from build123d import *

# Parameters (mm, degrees)
F1_DEPTH = 50.8


with BuildPart() as f1:
    # F0 (on Front) → F1 (new body)
    with BuildSketch(Plane.XZ):
        with BuildLine():
            Line((157.3511064053, 226.7855703831), (117.0178577304, 256.9078505039))
            Line((117.0178577304, 256.9078505039), (153.2667279243, 222.1906334162))
            Line((153.2667279243, 222.1906334162), (135.5471188815, 203.6892712114))
            ThreePointArc((135.5471188815, 203.6892712114), (124.4679795229, 189.3777542773), (142.5452232361, 188.4945183992))
            Line((142.5452232361, 188.4945183992), (157.3511064053, 188.4945183992))
            ThreePointArc((157.3511064053, 188.4945183992), (163.0913283676, 173.9439144731), (157.3511064053, 159.3933105469))
            ThreePointArc((157.3511064053, 159.3933105469), (133.5218764448, 146.628732852), (106.8485764131, 151.0221039559))
            ThreePointArc((106.8485764131, 151.0221039559), (81.4826477265, 155.0355463169), (59.0786326768, 142.4817354462))
            ThreePointArc((59.0786326768, 142.4817354462), (57.1778936646, 140.1694279188), (55.4591871163, 137.7187907169))
            ThreePointArc((55.4591871163, 137.7187907169), (49.1972996165, 115.7594263547), (56.2388920861, 94.0375274104))
            ThreePointArc((56.2388920861, 94.0375274104), (51.4005357949, 84.435997918), (44.5201359689, 76.1740878224))
            ThreePointArc((44.5201359689, 76.1740878224), (33.1757105593, 71.4588467738), (31.2459021807, 59.3260265887))
            ThreePointArc((31.2459021807, 59.3260265887), (28.0144474885, 44.7267728634), (21.5454995632, 31.2459263951))
            ThreePointArc((21.5454995632, 31.2459263951), (25.0258299967, 19.4454210796), (26.6509782523, 7.2501958348))
            Line((26.6509782523, 7.2501958348), (45.5412305892, 7.2501958348))
            ThreePointArc((45.5412305892, 7.2501958348), (43.9865002742, 15.1994537749), (37.8830172122, 20.52443102))
            ThreePointArc((37.8830172122, 20.52443102), (39.9724122876, 31.2459263951), (37.8830172122, 41.9674217701))
            ThreePointArc((37.8830172122, 41.9674217701), (43.3657124777, 53.2576823746), (51.4005357949, 62.8998577595))
            ThreePointArc((51.4005357949, 62.8998577595), (63.9434482796, 70.1826306752), (75.6635218859, 78.7268280983))
            ThreePointArc((75.6635218859, 78.7268280983), (79.7479003668, 78.2162845135), (83.8322788477, 78.7268280983))
            ThreePointArc((83.8322788477, 78.7268280983), (80.62219761, 70.8415194676), (75.6635218859, 63.9209523797))
            ThreePointArc((75.6635218859, 63.9209523797), (94.8811032097, 51.3116760169), (110.8912838002, 34.8197567898))
            Line((110.8912838002, 34.8197567898), (118.0389523506, 23.5877130181))
            ThreePointArc((118.0389523506, 23.5877130181), (122.7991958663, 28.8657998516), (124.165520072, 35.8408465981))
            ThreePointArc((124.165520072, 35.8408465981), (117.7349645729, 43.3549786498), (114.4651249051, 52.6889152825))
            ThreePointArc((114.4651249051, 52.6889152825), (101.2536184714, 56.1015596962), (93.0221304297, 66.9842362404))
            ThreePointArc((93.0221304297, 66.9842362404), (105.7958752022, 76.2573128263), (114.4651249051, 89.4483178854))
            ThreePointArc((114.4651249051, 89.4483178854), (137.6729881459, 85.3431639936), (161.1937859731, 86.8362394266))
            Line((161.1937859731, 86.8362394266), (161.1937859731, 60.947837063))
            add(Edge.make_bspline(
                [(161.1937859731, 60.947837063), (157.8993693687, 59.0561358776), (150.6323180509, 54.8832909577), (162.2144334117, 39.9763215602), (143.2040633117, 24.6385665246), (159.3573781955, 18.7003155427), (150.8482458466, 9.9391907933), (152.7499995265, 7.8050355296)],
                knots=[0, 0, 0, 0, 0.0779334272, 0.1719109278, 0.2757758884, 0.3531240541, 0.4319815568, 0.4319815568, 0.4319815568, 0.4319815568], degree=3))
            Line((152.7499995265, 7.8050355296), (173.171891931, 9.0224858617))
            ThreePointArc((173.171891931, 9.0224858617), (172.9779809567, 10.1232568284), (172.664853356, 11.1962196856))
            add(Edge.make_bspline(
                [(172.664853356, 11.1962196856), (171.3313436819, 12.7085104711), (168.5824067748, 14.597468285), (167.0453242097, 17.1912484114)],
                knots=[0.5736467919, 0.5736467919, 0.5736467919, 0.5736467919, 0.6257117477, 0.6257117477, 0.6257117477, 0.6257117477], degree=3))
            add(Edge.make_bspline(
                [(167.0453242097, 17.1912484114), (166.5426299969, 18.0395296218), (166.169553332, 18.9631972351), (165.9011092746, 19.9468993754)],
                knots=[0.6257117477, 0.6257117477, 0.6257117477, 0.6257117477, 0.6427392989, 0.6427392989, 0.6427392989, 0.6427392989], degree=3))
            ThreePointArc((165.9011092746, 19.9468993754), (164.2768081704, 31.0782012829), (167.0453242097, 41.9813914203))
            add(Edge.make_bspline(
                [(167.0453242097, 41.9813914203), (167.3962963394, 49.2992780507), (165.4846355858, 55.0477309675), (167.0453242097, 61.3542387283)],
                knots=[0.7506807864, 0.7506807864, 0.7506807864, 0.7506807864, 0.8611546748, 0.8611546748, 0.8611546748, 0.8611546748], degree=3))
            add(Edge.make_bspline(
                [(167.0453242097, 61.3542387283), (169.0068222846, 69.2803571375), (176.4531944079, 78.0879710988), (183.8995665312, 86.8955850601)],
                knots=[0.8611546748, 0.8611546748, 0.8611546748, 0.8611546748, 1, 1, 1, 1], degree=3))
            ThreePointArc((183.8995665312, 86.8955850601), (200.6813055662, 83.248064902), (217.7208593273, 85.3892738977))
            ThreePointArc((217.7208593273, 85.3892738977), (229.8786920932, 81.8087152157), (231.4277632013, 69.2296183983))
            Line((231.4277632013, 69.2296183983), (228.5562352695, 63.4104087949))
            Line((228.5562352695, 63.4104087949), (231.4277632013, 57.001966241))
            Line((231.4277632013, 57.001966241), (221.0727564471, 52.3620415043))
            Line((221.0727564471, 52.3620415043), (222.7011620998, 44.7454368664))
            Line((222.7011620998, 44.7454368664), (237.3357014598, 47.8742544631))
            Line((237.3357014598, 47.8742544631), (240.5703216791, 63.4104087949))
            Line((240.5703216791, 63.4104087949), (240.5703216791, 81.790111959))
            ThreePointArc((240.5703216791, 81.790111959), (237.5070340931, 96.5959839523), (222.7011620998, 99.6592715383))
            Line((222.7011620998, 99.6592715383), (208.9163959026, 107.8280285001))
            ThreePointArc((208.9163959026, 107.8280285001), (216.2226754166, 127.6019199845), (215.5535072088, 148.6718207598))
            ThreePointArc((215.5535072088, 148.6718207598), (218.0854842896, 143.9483475476), (222.190618515, 140.503063798))
            ThreePointArc((222.190618515, 140.503063798), (220.0514151702, 151.3432226251), (215.5535072088, 161.4354997873))
            Line((215.5535072088, 161.4354997873), (229.0830209851, 152.8838410974))
            Line((229.0830209851, 152.8838410974), (214.0218615532, 172.6675480604))
            Line((214.0218615532, 172.6675480604), (219.6378856897, 172.6675480604))
            Line((219.6378856897, 172.6675480604), (208.4058374166, 184.6981031667))
            Line((208.4058374166, 184.6981031667), (213.5113179684, 186.4523291588))
            Line((213.5113179684, 186.4523291588), (208.4058374166, 201.3112651118))
            Line((208.4058374166, 201.3112651118), (213.5113179684, 201.7687410116))
            Line((213.5113179684, 201.7687410116), (200.6355195315, 214.0218764544))
            Line((200.6355195315, 214.0218764544), (208.4058374166, 213.5113328695))
            ThreePointArc((208.4058374166, 213.5113328695), (200.6355195315, 219.8232430535), (191.0472214222, 222.7011919022))
            ThreePointArc((191.0472214222, 222.7011919022), (182.6973201136, 228.8132361759), (172.5500786904, 226.7855703831))
            Line((172.5500786904, 226.7855703831), (167.7524379956, 231.3804924488))
            Line((167.7524379956, 231.3804924488), (167.7524379956, 226.7855703831))
            Line((167.7524379956, 226.7855703831), (161.0753406305, 231.77226012))
            Line((161.0753406305, 231.77226012), (157.3511064053, 226.7855703831))
        make_face()
        with BuildLine():
            ThreePointArc((55.4591871163, 137.7187907169), (57.1778936646, 140.1694279188), (59.0786326768, 142.4817354462))
            ThreePointArc((59.0786326768, 142.4817354462), (39.0356978447, 161.9894984881), (18.9927630126, 142.4817354462))
            ThreePointArc((18.9927630126, 142.4817354462), (15.5809128086, 125.4101537656), (18.9927630126, 108.3385720849))
            Line((18.9927630126, 108.3385720849), (22.309999913, 97.1100777388))
            Line((22.309999913, 97.1100777388), (22.309999913, 84.7518071532))
            Line((22.309999913, 84.7518071532), (33.4528027138, 104.264870286))
            Line((33.4528027138, 104.264870286), (33.4528027138, 86.6916491587))
            Line((33.4528027138, 86.6916491587), (36.9130928491, 112.466349486))
            Line((36.9130928491, 112.466349486), (43.123934418, 97.1100777388))
            ThreePointArc((43.123934418, 97.1100777388), (41.9493193566, 113.4261599819), (37.8830172122, 129.2710155249))
            ThreePointArc((37.8830172122, 129.2710155249), (41.7069327363, 143.8231946906), (55.4591871163, 137.7187907169))
        make_face()
    extrude(amount=F1_DEPTH)


solid = f1.part
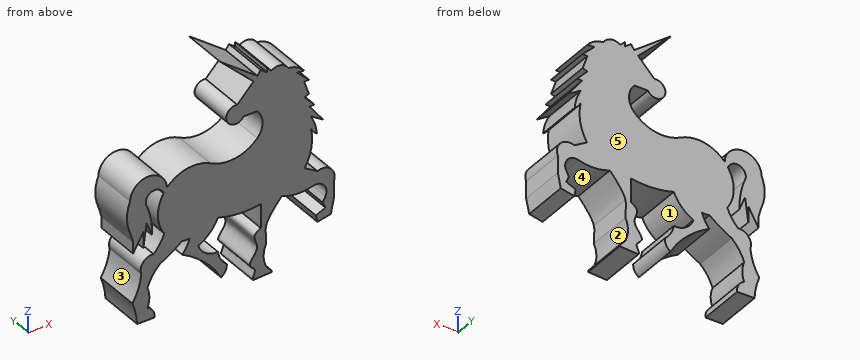
For this review, take the finished solid that the model builds, in its own axes (mm). Face numbers are marked on the shaded views. A direction names the side the tool comes from. Coordinates: 2 decimals unless noted, no trailing zeros. Loops run counter-clockwise (first coordinate to the right, second up) from the corner with the lowest first, then second, coordinate; pieces in that order, holes last. Notation, with made-up numbers: (44.25, 1.5) -> (87.25, 1.5) arc R35 ccw to (87.25, 40.5) -> close; hole circle Ø7 at (-32.75, -10.75). An arc over 180 degrees is marked (long way). Write each question's results on one line, items separated by ' | '.
Q1. Add section B-B, the plane z = 217.5. State the section outline as (x, y) points, then the cut area to 3 significant figures.
Taken from the geometry:
outline: (148.77, -50.8) -> (204.26, -50.8) -> (204.26, 0) -> (148.77, 0) -> close | area: 2,820 mm²
Q2. For pin 1 Ø1.5 at (x, y) = (192, -27) entering from +Z; pin 2 Ø2.5 at (y, z) = (-36.5, 230) entering from -X; pin 3 Ø3.5 at (y, z) = (-33, 89) entering from -X, all flat-tipped, find the tip position at first contact; note any pin that passes through.
Taken from the geometry:
pin 1: z = 222.68 | pin 2: x = 143.81 | pin 3: x = 22.31
Q3. Mouldability with a two-part tool opening along X and no side actions: class the marked faces 3, 4 and 5 as +X half, -X half, draft (parallel to the pull), parting line (faces both ways), or undercut.
Taken from the geometry:
face 3: -X half | face 4: undercut | face 5: draft
Q4. Machinability: for the marked faces 1 and 2, which of the approach directions +Z, -Z, +X, -X, +Y, -Y give a long, thin tool a straight path to every point of the face, cutting with its end or side? Answer none if there is none.
Taken from the geometry:
face 1: +Y, -Y | face 2: +X, +Y, -Y
Q5. To check wall thickness, follow line 1 along X through (y, z) = (-43.5, 50); line 2 along X through (y, z) = (-33, 24); line 3 along X through (y, z) = (-9, 228) (3 decimals). State the ranges of each line that lie inside material, in increasing order. Write a range as [from, to].
Taken from the geometry:
line 1: [29.59, 41.43], [96.44, 115.02], [155.08, 166.76], [221.58, 237.78] | line 2: [23.92, 39.04], [117.78, 118.65], [149.6, 164.79] | line 3: [147.201, 155.725], [158.258, 166.126], [167.752, 171.282], [174.692, 185.163]
Q6. Add section C-C, the plane x = 196. State the section outline as (y, z) points, then the cut area to 3 significant figures.
Taken from the geometry:
outline: (-50.8, 83.67) -> (0, 83.67) -> (0, 221.73) -> (-50.8, 221.73) -> close | area: 7,010 mm²
Q7. Add section A-A, the plane x = 145.5. State the section outline as (y, z) points.
Taken from the geometry:
outline: (-50.8, 85.22) -> (0, 85.22) -> (0, 150.53) -> (-50.8, 150.53) -> close; (-50.8, 188.49) -> (0, 188.49) -> (0, 214.08) -> (-50.8, 214.08) -> close; (-50.8, 229.63) -> (0, 229.63) -> (0, 235.64) -> (-50.8, 235.64) -> close
